Input: dimensioned drawing with shaded views. Units: mm. Origin: part minimum x, y, z. A direction names the side the tool comes from. Give positions to 0.01 mm unless a question says otherwise; leave off trailing zeros. Write each loop counter-clockwise with the first axis right and the second up, starting at its lowest first coordinate (ties: lowest second). Pieces come first, ordered by that corner, then holes.
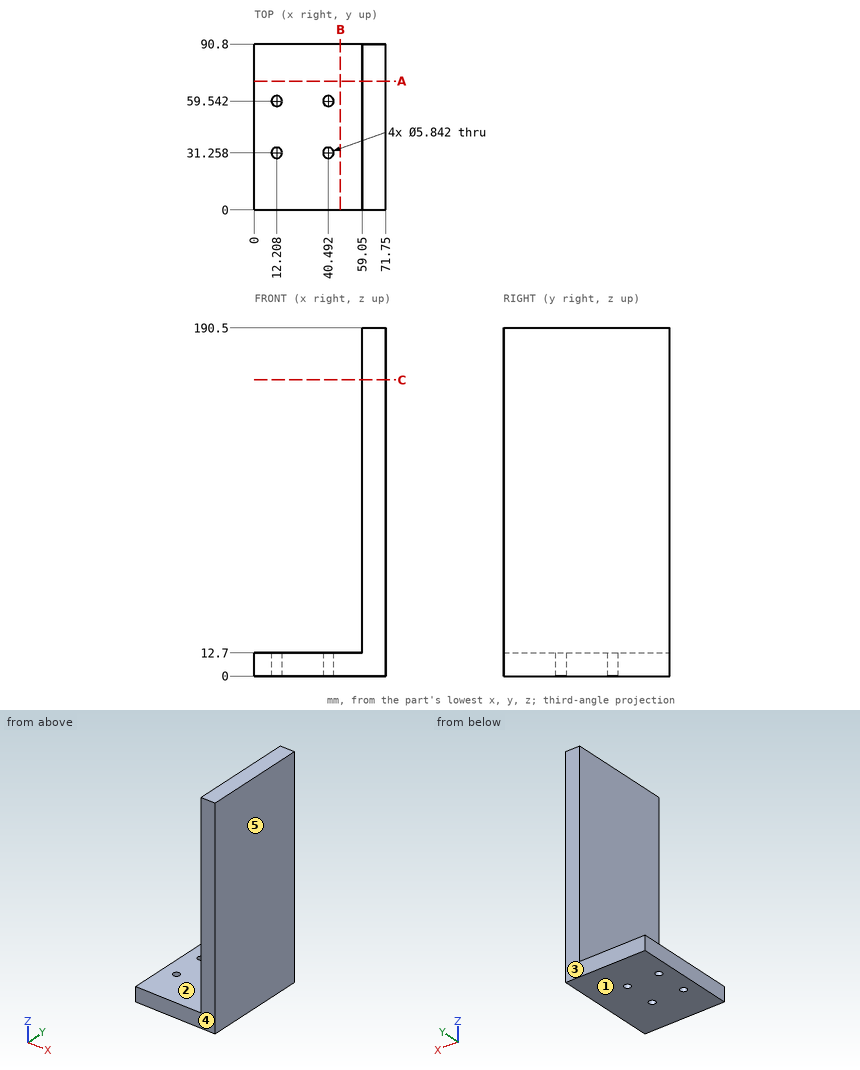
Item 1: Section C-C (z = 162). Return loops of the section in (x, y).
Item 2: Set-up query: the marked faces 1 and 2. Return all of +Z, -Z, +X, -X, +Y, -Y with unobstructed straight access to the full face (end or side cutting, diameter ignored); none if empty.
Item 3: Pin query (flat end, axial travel): pin 1 (9.5 mm diameter, centred on x = 40.49, y = 31.26, fed in from +Z); pin 2 (1.5 mm diameter, centred on y = 69, z = 155, fed in from -X). Return the tip coordinate at first contact, or that it passes through.
Item 4: Ray query, line 1 (X direction, y = 58, z = 12); line 2 (Z direction, x = 17.5, y = 24); line 3 (X direction, y = 55.5, z = 131). Return the intervals inside material, ascending.
Item 5: Mould query, pull axis Y, two halves, no side actions, for the marked faces 3, 4 and 5. Classes: +Y half, -Y half, draft (parallel to the pull), parting line (faces both ways), or undercut.
Item 6: Section A-A (y = 70.5). Return loops of the section in (x, z).
Item 7: Section B-B (x = 47). Return loops of the section in (y, z).
Solved:
1. outline: (59.05, 0) - (71.75, 0) - (71.75, 90.8) - (59.05, 90.8) - close
2. face 1: -Z, +X, -X, +Y, -Y
2. face 2: +Z, -X, +Y, -Y
3. pin 1: stops at z = 12.7
3. pin 2: stops at x = 59.05
4. line 1: x = 0 to 9.73, 14.69 to 38.01, 42.97 to 71.75
4. line 2: z = 0 to 12.7
4. line 3: x = 59.05 to 71.75
5. face 3: +Y half
5. face 4: -Y half
5. face 5: draft
6. outline: (0, 0) - (71.75, 0) - (71.75, 190.5) - (59.05, 190.5) - (59.05, 12.7) - (0, 12.7) - close
7. outline: (0, 0) - (90.8, 0) - (90.8, 12.7) - (0, 12.7) - close
